Autodesk Inventor part; units mm, degrees
ref_plane "YZ Plane" through (0, 0, 0) normal (1, 0, 0) x (0, 1, 0)
ref_plane "XZ Plane" through (0, 0, 0) normal (0, 1, 0) x (-1, 0, 0)
ref_plane "XY Plane" through (0, 0, 0) normal (0, 0, 1) x (1, 0, 0)
sketch "Sketch1" plane through (0, 0, 0) normal (0, 0, 1) x (1, 0, 0)
  line L0 (82.5, -24.5) -> (-82.5, -24.5)
  line L1 (-82.5, -24.5) -> (-82.5, 24.5)
  line L2 (-82.5, 24.5) -> (82.5, 24.5)
  line L3 (82.5, 24.5) -> (82.5, -24.5)
  circle A0 centre (-28.2, -14.95) radius 3.1
  circle A1 centre (6, -14.95) radius 3.1
  circle A2 centre (40.2, -14.95) radius 3.1
  circle A3 centre (57.3, -14.95) radius 3.1
  circle A4 centre (23.1, -14.95) radius 3.1
  circle A5 centre (-11.1, -14.95) radius 3.1
  circle A6 centre (-45.3, -14.95) radius 3.1
  line L4 (-25.1, 0.4) -> (-31.3, 0.4)
  line L5 (-31.3, 0.4) -> (-31.3, 13.9)
  line L6 (-31.3, 13.9) -> (-25.1, 13.9)
  line L7 (-25.1, 13.9) -> (-25.1, 0.4)
  line L8 (9.1, 0.4) -> (2.9, 0.4)
  line L9 (2.9, 0.4) -> (2.9, 13.9)
  line L10 (2.9, 13.9) -> (9.1, 13.9)
  line L11 (9.1, 13.9) -> (9.1, 0.4)
  line L12 (43.3, 0.4) -> (37.1, 0.4)
  line L13 (37.1, 0.4) -> (37.1, 13.9)
  line L14 (37.1, 13.9) -> (43.3, 13.9)
  line L15 (43.3, 13.9) -> (43.3, 0.4)
  line L16 (54.2, 0.4) -> (54.2, 13.9)
  line L17 (54.2, 13.9) -> (60.4, 13.9)
  line L18 (60.4, 13.9) -> (60.4, 0.4)
  line L19 (60.4, 0.4) -> (54.2, 0.4)
  line L20 (26.2, 0.4) -> (20, 0.4)
  line L21 (20, 0.4) -> (20, 13.9)
  line L22 (20, 13.9) -> (26.2, 13.9)
  line L23 (26.2, 13.9) -> (26.2, 0.4)
  line L24 (-8, 0.4) -> (-14.2, 0.4)
  line L25 (-14.2, 0.4) -> (-14.2, 13.9)
  line L26 (-14.2, 13.9) -> (-8, 13.9)
  line L27 (-8, 13.9) -> (-8, 0.4)
  line L28 (-42.2, 0.4) -> (-48.4, 0.4)
  line L29 (-48.4, 0.4) -> (-48.4, 13.9)
  line L30 (-48.4, 13.9) -> (-42.2, 13.9)
  line L31 (-42.2, 13.9) -> (-42.2, 0.4)
  arc A7 (73.05, -22.25) -> (80.25, -15.05) centre (73.05, -15.05) ccw
  line L32 (80.25, -15.05) -> (80.25, 15.05)
  arc A8 (80.25, 15.05) -> (73.05, 22.25) centre (73.05, 15.05) ccw
  line L33 (73.05, 22.25) -> (-73.05, 22.25)
  arc A9 (-73.05, 22.25) -> (-80.25, 15.05) centre (-73.05, 15.05) ccw
  line L34 (-80.25, 15.05) -> (-80.25, -15.05)
  arc A10 (-80.25, -15.05) -> (-73.05, -22.25) centre (-73.05, -15.05) ccw
  line L35 (-73.05, -22.25) -> (73.05, -22.25)
  line L36 (-73.05, -22.25) -> (73.05, -22.25)
  point P0 (0, 0)
  dimension "d0" = 2.25
  dimension "d1" = 2.25
  dimension "d2" = 2.25
  dimension "d3" = 2.25
extrude "Extrusion1" add sketch "Sketch1" along normal blind 2 contours L0 L1 L2 L3 | L35 A10 L34 A9 L33 A8 L32 A7
sketch "Sketch2" plane through (0, 0, 0) normal (0, 0, -1) x (-1, 0, 0)
  line L0 (-82.5, -24.5) -> (-82.5, 24.5)
  line L1 (-82.5, -24.5) -> (-80.5, -24.5)
  line L2 (-80.5, -24.5) -> (-80.5, 24.5)
  line L3 (-80.5, 24.5) -> (-82.5, 24.5)
  line L4 (-82.5, 24.5) -> (-82.5, -24.5)
  line L5 (82.5, 24.5) -> (-82.5, 24.5)
  line L6 (82.5, 24.5) -> (82.5, -24.5)
  line L7 (-82.5, -24.5) -> (82.5, -24.5)
  line L8 (82.5, -24.5) -> (82.5, -22.5)
  line L9 (82.5, -22.5) -> (-82.5, -22.5)
  line L10 (-82.5, -22.5) -> (-82.5, -24.5)
  line L11 (82.5, -24.5) -> (-82.5, -24.5)
  line L12 (-82.5, 24.5) -> (82.5, 24.5)
  line L13 (82.5, -24.5) -> (80.5, -24.5)
  line L14 (80.5, -24.5) -> (80.5, 24.5)
  line L15 (80.5, 24.5) -> (82.5, 24.5)
  line L16 (82.5, 24.5) -> (82.5, -24.5)
  line L17 (82.5, 24.5) -> (-82.5, 24.5)
  line L18 (-82.5, 24.5) -> (-82.5, 22.5)
  line L19 (-82.5, 22.5) -> (82.5, 22.5)
  line L20 (82.5, 22.5) -> (82.5, 24.5)
  point P0 (0, 0)
  dimension "d6" = 2
  dimension "d7" = 2
  dimension "d8" = 2
  dimension "d9" = 2
extrude "Extrusion2" add sketch "Sketch2" along normal blind 20 contours L0 L9 L2 L1 | L0 L19 L2 L9 | L2 L9 L14 L7 | L0 L3 L2 L19 | L14 L9 L6 L7 | L2 L5 L14 L19 | L14 L19 L6 L9 | L14 L5 L6 L19
sketch "Sketch3" plane through (-82.5, -24.5, 2) normal (-1, 0, 0) x (0, 0, 1)
  circle A0 centre (-15.3, 16.55) radius 5.3 construction
  circle A1 centre (-16.35, 35.4) radius 2.25 construction
  arc A2 (-16.35, 32.15) -> (-16.35, 38.65) centre (-16.35, 35.4) ccw
  arc A3 (-15.3, 10.25) -> (-15.3, 22.85) centre (-15.3, 16.55) ccw
  line L0 (-16.35, 38.65) -> (-22, 38.65)
  line L1 (-22, 2) -> (-22, 47)
  line L2 (-16.35, 32.15) -> (-22, 32.15)
  line L3 (-15.3, 22.85) -> (-22, 22.85)
  line L4 (-15.3, 10.25) -> (-22, 10.25)
  line L5 (-22, 10.25) -> (-22, 22.85)
  line L6 (-22, 32.15) -> (-22, 38.65)
  arc A4 (-15.3, 22.85) -> (-15.3, 10.25) centre (-15.3, 16.55) ccw construction
  arc A5 (-16.35, 38.65) -> (-16.35, 32.15) centre (-16.35, 35.4) ccw construction
  point P0 (-2, 24.5)
  dimension "d12" = 1
  dimension "d13" = 1
extrude "Extrusion3" cut sketch "Sketch3" against normal blind 20
sketch "Sketch4" plane through (82.5, -24.5, 2) normal (1, 0, 0) x (0, 0, -1)
  line L0 (18.25, 17.75) -> (11.45, 17.75)
  line L1 (11.45, 17.75) -> (11.45, 31.25)
  line L2 (11.45, 31.25) -> (18.25, 31.25)
  line L3 (18.25, 31.25) -> (18.25, 17.75)
  line L4 (25.6, 9.45) -> (2, 9.45)
  line L5 (25.6, 39.55) -> (25.6, 9.45)
  line L6 (2, 39.55) -> (25.6, 39.55)
  line L7 (2, 9.45) -> (2, 39.55)
  line L8 (10.45, 16.75) -> (22, 16.75)
  line L9 (22, 16.75) -> (22, 32.25)
  line L10 (22, 32.25) -> (10.45, 32.25)
  line L11 (10.45, 32.25) -> (10.45, 16.75)
  line L12 (22, 49) -> (22, 0)
  point P0 (2, 24.5)
  dimension "d16" = 1
  dimension "d17" = 1
  dimension "d19" = 1
extrude "Extrusion4" cut sketch "Sketch4" against normal blind 20 contours L0 L1 L2 L3 | L8 L11 L10 L9
chamfer "Chamfer1" distance 2 angle 45 35 edges at (-45.3, 13.9, 2) (-48.4, 7.15, 2) (-45.3, 0.4, 2) (-42.2, 7.15, 2) (-31.3, 7.15, 2) (-28.2, 13.9, 2) (-25.1, 7.15, 2) (-28.2, 0.4, 2) (-14.2, 7.15, 2) (-11.1, 13.9, 2) (-8, 7.15, 2) (-11.1, 0.4, 2) (2.9, 7.15, 2) (6, 13.9, 2) (9.1, 7.15, 2) (6, 0.4, 2) (26.2, 7.15, 2) (23.1, 13.9, 2) (20, 7.15, 2) (23.1, 0.4, 2) (40.2, 0.4, 2) (37.1, 7.15, 2) (40.2, 13.9, 2) (43.3, 7.15, 2) (54.2, 7.15, 2) (57.3, 13.9, 2) (60.4, 7.15, 2) (57.3, 0.4, 2) (54.2, -14.95, 2) (37.1, -14.95, 2) (20, -14.95, 2) (2.9, -14.95, 2) (-14.2, -14.95, 2) (-31.3, -14.95, 2) (-48.4, -14.95, 2)
equation "\"d1\" = d0"
equation "\"d2\" = d0"
equation "\"d3\" = d0"
equation "\"d17\" = d16"
equation "\"d19\" = d16"
properties part number "cover"
Read the model definition and answer for the solid it produces. Units are mm, in the model's axes. A direction names the side the tool comes from. Coordinates: 2 decimals unless noted, no trailing zeros. Loops run counter-clockwise (first coordinate to the right, second up) from the corner with the lowest first, then second, coordinate; pieces in that order, holes last. Notation, with made-up numbers: (0, 40.5) - (47, 40.5) arc R32 cw to (47, 73.5) - close; hole circle Ø4 at (-34, 84). An arc over 180 degrees is marked (long way). Answer in a Markdown table with one row per item.
1. Given pin 1 (1 mm diameter, centred on x = -16, y = 13.5, fed in from -Z); pin 2 (0.6 mm diameter, centred on x = 81, y = 0, fed in from -Z); pin 3 (12 mm diameter, centred on x = -43.5, y = -1, fed in from +Z); pin 4 (8 mm diameter, centred on x = -45.3, y = -14.95, fed in from +Z), each flat-ended and moving along its own axis, determine where each tip first touches the part or whether it passes through.
Conclusion:
| item | result |
|---|---|
| pin 1 | stops at z = 0 |
| pin 2 | stops at z = -8.45 |
| pin 3 | stops at z = 2 |
| pin 4 | stops at z = 0.9 |
2. Find section B-B, the plane x = 57.3. Count the separate pieces of the cut face and the enclosed holes in it, then the cut area to 3 significant figures.
Conclusion:
| item | result |
|---|---|
| separate pieces | 3 |
| enclosed holes | 0 |
| area | 131 mm² |
3. Determine the mould class of faces 1 (the face through (0, 24, -20)), 2 (the face through (-80.5, 0, -10)), 3 (the face through (-1, 24.5, -9)) for opening direction Y: +Y half, -Y half, draft (parallel to the pull), parting line (faces both ways), or undercut.
Conclusion:
| item | result |
|---|---|
| face 1 | draft |
| face 2 | undercut |
| face 3 | +Y half |
4. Find section D-D, the plane y = 20. Write down the section's boundary in (x, z).
Conclusion:
| item | result |
|---|---|
| outline | (-82.5, -20) - (-80.5, -20) - (-80.5, 0) - (80.5, 0) - (80.5, -20) - (82.5, -20) - (82.5, 2) - (-82.5, 2) - close |
5. Find section A-A, the plane z = -3.75. Write down the section's boundary in (x, y), then the cut area to 3 significant figures.
Conclusion:
| item | result |
|---|---|
| outline | (-82.5, -24.5) - (82.5, -24.5) - (82.5, 24.5) - (-82.5, 24.5) - close; hole (-80.5, -22.5) - (80.5, -22.5) - (80.5, 22.5) - (-80.5, 22.5) - close |
| area | 840 mm² |
6. Which of the six approach directions +Z, -Z, +X, -X, +Y, -Y give full straight-line access (tool end or side, diameter ignored) to faces 4 (the face through (-1, 0, 2)), 5 (the face through (80.5, 0, -8)), 6 (the face through (-81.5, 10.8, -11.1))?
Conclusion:
| item | result |
|---|---|
| face 4 | +Z, +X, -X, +Y, -Y |
| face 5 | -Z |
| face 6 | -Z, -X |
7. Straight lines are drawn through the part: line 1 (X direction, y = 21, z = -1.5); line 2 (Y direction, x = 60.5, z = -14); line 3 (X direction, y = -14, z = -17.5). For each, find the intervals that lie inside material, in ascending order.
Conclusion:
| item | result |
|---|---|
| line 1 | x = -82.5 to -80.5, 80.5 to 82.5 |
| line 2 | y = -24.5 to -22.5, 22.5 to 24.5 |
| line 3 | x = 80.5 to 82.5 |
8. Find section C-C, the plane z = -15.75. Write down the section's boundary in (x, y), then the cut area to 3 significant figures.
Conclusion:
| item | result |
|---|---|
| outline | (-82.5, -24.5) - (82.5, -24.5) - (82.5, -7.75) - (80.5, -7.75) - (80.5, -22.5) - (-80.5, -22.5) - (-80.5, -14.25) - (-82.5, -14.25) - close; (-82.5, -1.65) - (-80.5, -1.65) - (-80.5, 7.65) - (-82.5, 7.65) - close; (-82.5, 14.15) - (-80.5, 14.15) - (-80.5, 22.5) - (80.5, 22.5) - (80.5, 7.75) - (82.5, 7.75) - (82.5, 24.5) - (-82.5, 24.5) - close |
| area | 771 mm² |
